Geometry: final body of the model. Coordinates: model frame, mm. Face numbers are marked on the shaded views. A direction names the side the tool comes from. Coordinates: 2 decimals unless noted, no trailing zeros. Order: outer loops, then holes, each group sorted by start corner. A loop starts at its lowest first (then second) coordinate and runs counter-clockwise, first axis right, second up. Notation, with made-up numbers: (20, 23) -> (44, 23) arc R15 cw to (44, 52) -> close; hole circle Ø2 at (17, 51). An arc over 180 degrees is marked (long way). Use CSV: the item, a comma, the result in double quotes. Start each with the question number.
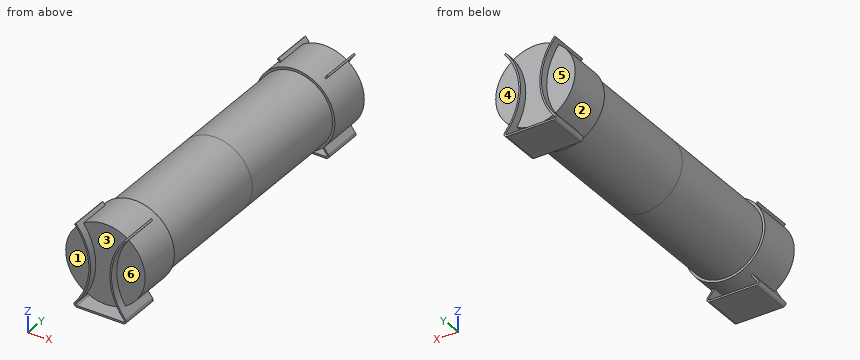
from build123d import *

# Parameters (mm, degrees)
F1_DEPTH = 17.5
F3_R     = 17
F4_DEPTH = 19.05
F5_R     = 16
F6_DEPTH = 52.07


with BuildPart() as f1:
    # F0 (on Front) → F1 (new body)
    with BuildSketch(Plane.XZ):
        with BuildLine():
            Line((-19.309289, 16.501859), (-19.833244, 16.992354))
            ThreePointArc((-19.833244, 16.992354), (-26.117, 0), (-19.833244, -16.992354))
            Line((-19.833244, -16.992354), (-19.309289, -16.501859))
            ThreePointArc((-19.309289, -16.501859), (-25.4, 0), (-19.309289, 16.501859))
        make_face()
        with BuildLine():
            Line((-19.309289, -16.501859), (-19.833244, -16.992354))
            ThreePointArc((-19.833244, -16.992354), (-19.866141, -17.4713), (-20.287276, -17.701772))
            Line((-20.287276, -17.701772), (-40.180276, -17.701772))
            Line((-40.180276, -17.701772), (-40.180276, -18.466977))
            Line((-40.180276, -18.466977), (-20.287276, -18.466977))
            ThreePointArc((-20.287276, -18.466977), (-19.214267, -17.775067), (-19.309289, -16.501859))
        make_face()
        with BuildLine():
            Line((-40.180276, -18.466977), (-40.180276, -17.701772))
            ThreePointArc((-40.180276, -17.701772), (-40.60141, -17.4713), (-40.634307, -16.992354))
            Line((-40.634307, -16.992354), (-41.158262, -16.501859))
            ThreePointArc((-41.158262, -16.501859), (-41.253285, -17.775067), (-40.180276, -18.466977))
        make_face()
        with BuildLine():
            Line((-41.158262, -16.501859), (-40.634307, -16.992354))
            ThreePointArc((-40.634307, -16.992354), (-34.350551, 0), (-40.634307, 16.992354))
            Line((-40.634307, 16.992354), (-41.158262, 16.501859))
            ThreePointArc((-41.158262, 16.501859), (-35.067551, 0), (-41.158262, -16.501859))
        make_face()
    extrude(amount=F1_DEPTH)

    # F3 (on offset) → F4 (join)
    with BuildSketch(Plane.XZ.offset(14.1)):
        with Locations((-30.233776, 1.533023)):
            Circle(F3_R)
    extrude(amount=-F4_DEPTH)

    # F5 (on face) → F6 (join)
    with BuildSketch(Plane(origin=(0, 4.95, 0), x_dir=(-1, 0, 0), z_dir=(0, 1, 0))):
        with Locations((30.233776, 1.533023)):
            Circle(F5_R)
    extrude(amount=F6_DEPTH)

    # F8: F1 across plane


with BuildPart() as f1_1:
    add(f1.part)
    add(f1.part.mirror(Plane.XZ.offset(-57.02)))


solid = f1_1.part
(1) Section D-D (x = -16). Return loops of the section in (y, z).
(2) Section A-A (x = -32). Return loops of the section in (y, z), then the cut area to 3 significant figures.
(3) Access query for the marked faces 4, 5 and 6. Directions: +Z, -Z, +X, -X, +Y, -Y. A direction counts if a zero-diameter tool reaches every point of the face in a straight line with its end or side. Return the directions, or none.
(4) Section C-C (z = -7). Return loops of the section in (x, y), then the cut area to 3 significant figures.
(5) Section B-B (y = 116). Return loops of the section in (x, z).
(6) First-contact query: pin 1 (3 mm diameter, centred on x = -31.5, y = 91.5, fed in from -Z); pin 2 (5 mm diameter, centred on y = 97.5, z = -5, fed in from -X); pin 3 (10 mm diameter, centred on y = 41.5, z = 11, fed in from -X). Flat tips, straight axial feed; report the tip coordinate or a pass-through.
(7) Line query: line 1 (X direction, y = -10, z = 16); line 2 (Y direction, x = -24, z = -11.5); line 3 (Z direction, x = -31.5, y = 119). Output: solid intervals per line, ascending. Write a range as from..to.
(8) Mould query, pull axis X, two halves, no side actions, for the marked faces 1, 2 and 3. Classes: pulls with the +X half, pulls with the -X half, needs draft (parallel to the pull), parting line crosses it, or undercut.
Check sheet entries:
1,outline,"(-14.1, -7.76) -> (4.95, -7.76) -> (4.95, -5.77) -> (109.09, -5.77) -> (109.09, -7.76) -> (128.14, -7.76) -> (128.14, 10.83) -> (109.09, 10.83) -> (109.09, 8.84) -> (4.95, 8.84) -> (4.95, 10.83) -> (-14.1, 10.83) -> close"
2,outline,"(-17.5, -18.47) -> (0, -18.47) -> (0, -17.7) -> (-17.5, -17.7) -> close; (-14.1, -15.37) -> (4.95, -15.37) -> (4.95, -14.37) -> (109.09, -14.37) -> (109.09, -15.37) -> (128.14, -15.37) -> (128.14, 18.44) -> (109.09, 18.44) -> (109.09, 17.44) -> (4.95, 17.44) -> (4.95, 18.44) -> (-14.1, 18.44) -> close; (114.04, -18.47) -> (131.54, -18.47) -> (131.54, -17.7) -> (114.04, -17.7) -> close"
2,area,"4,630 mm^2"
3,face 4,"+X, +Y"
3,face 5,"-X, +Y"
3,face 6,"+X, -Y"
4,outline,"(-44.94, -14.1) -> (-36.05, -14.1) -> (-36.05, -17.5) -> (-35.31, -17.5) -> (-35.31, -14.1) -> (-25.16, -14.1) -> (-25.16, -17.5) -> (-24.42, -17.5) -> (-24.42, -14.1) -> (-15.53, -14.1) -> (-15.53, 4.95) -> (-16.7, 4.95) -> (-16.7, 109.09) -> (-15.53, 109.09) -> (-15.53, 128.14) -> (-24.42, 128.14) -> (-24.42, 131.54) -> (-25.16, 131.54) -> (-25.16, 128.14) -> (-35.31, 128.14) -> (-35.31, 131.54) -> (-36.05, 131.54) -> (-36.05, 128.14) -> (-44.94, 128.14) -> (-44.94, 109.09) -> (-43.77, 109.09) -> (-43.77, 4.95) -> (-44.94, 4.95) -> close"
4,area,"3,950 mm^2"
5,outline,"(-41.16, -16.5) arc R1.25 ccw to (-40.18, -18.47) -> (-20.29, -18.47) arc R1.25 ccw to (-19.31, -16.5) arc R25.4 cw to (-21.71, -13.18) arc R17 ccw to (-20.27, 15.31) arc R25.4 cw to (-19.31, 16.5) -> (-19.83, 16.99) arc R26.12 ccw to (-20.86, 15.72) arc R17 ccw to (-39.61, 15.72) arc R26.12 ccw to (-40.63, 16.99) -> (-41.16, 16.5) arc R25.4 cw to (-40.2, 15.31) arc R17 ccw to (-38.75, -13.18) arc R25.4 cw to start; hole (-40.63, -16.99) arc R0.5 ccw to (-40.18, -17.7) -> (-20.29, -17.7) arc R0.5 ccw to (-19.83, -16.99) arc R26.12 cw to (-22.34, -13.52) arc R17 cw to (-38.13, -13.52) arc R26.12 cw to start"
6,pin 1,"stops at z = -14.47"
6,pin 2,"stops at x = -45.72"
6,pin 3,"stops at x = -45.6"
7,line 1,"x = -40.74..-39.83, -39.16..-21.31, -20.64..-19.73"
7,line 2,"y = -14.1..128.14"
7,line 3,"z = -18.47..-17.7, -15.42..18.49"
8,face 1,"needs draft"
8,face 2,"undercut"
8,face 3,"undercut"
